Can you work these out from the model? Positions are in its coordinate system, mm. A direction names the side the tool comes from. Coordinates: 2 decimals unless noted, no trailing zeros. Order: outer loops, then holes, each group sorted by start corner. A loop starts at its lowest first (then second) coordinate and runs counter-clockwise, first axis right, second up. Notation, with made-up numbers: (37, -4) - (71, -4) arc R20 ccw to (71, 25) - close; hole circle Ø1 at (52.25, 71.25). An arc over 180 degrees is marked (long way). Use a Markdown table: item, result. Add a question column.
(1) I want a section at B-B (y = -5). List the corners of the cut face in (x, z) for me, and give its area (3 significant figures).
(2) If I drill on L1, parallel to Y at x = 16.5, z = -2; L2, parallel to Z at x = 3.5, y = 1.5; L3, parallel to Y at x = 6.5, z = -8.5, over which ranges is the centre line in solid material (lowest first)? Write a range as [from, to].
(3) On a 3-axis mill with a long thin cutter (end or side, diameter ignored), from which of +Z, -Z, +X, -X, +Y, -Y can I reach the whole of each face in a straight line? I mean faces 1 (the flat face through (16, -1, -6)), 2 (the cylindrical face through (0.8, -0.8, -5.6)), 3 (the flat face through (16, 0, -2)), 4 (the cylindrical face through (31.13, -0.84, -5.65)). Say none if no direction works.
(4) I want a section at A-A (x = 8). List the corners of the cut face in (y, z) for me, and give its area (3 significant figures).
(5) I want a section at C-C (z = -3.5). List the corners of the cut face in (x, y) for me, and give its area (3 significant figures).
(6) I want a section at D-D (y = 1). List the corners of the cut face in (x, z) for me.
(7) For pin 1 Ø1.4 at (x, z) = (10.5, -3.5) entering from -Y; pin 2 Ø4 at (x, y) = (18.5, -4.5) entering from +Z; pin 3 Ø2.5 at (x, z) = (23, -8.5) entering from +Y, each with a flat end and sliding along its axis, tell me the tip position at first contact or that it passes through.
```python
from build123d import *
from build123d.topology import SkipClean

# Parameters (mm, degrees)
BOSS_EXTRUDE1_DEPTH = 2
BOSS_EXTRUDE2_START = -7.6
BOSS_EXTRUDE2_DEPTH = 7.6
BOSS_EXTRUDE3_DEPTH = 2
SKETCH5_W           = 32
SKETCH5_H           = 4.6
CUT_EXTRUDE1_DEPTH  = 34.990586932


with BuildPart() as part:
    # Sketch1 → Boss-Extrude1 (new body)
    with BuildSketch(Plane(origin=(0, 0, 0), x_dir=(1, 0, 0), z_dir=(0, 1, 0))):
        with BuildLine():
            Line((2, 0), (30, 0))
            ThreePointArc((30, 0), (31.414213562, 0.585786438), (32, 2))
            Line((32, 2), (32, 4))
            ThreePointArc((32, 4), (31.414213562, 5.414213562), (30, 6))
            Line((30, 6), (2, 6))
            ThreePointArc((2, 6), (0.585786438, 5.414213562), (0, 4))
            Line((0, 4), (0, 2))
            ThreePointArc((0, 2), (0.585786438, 0.585786438), (2, 0))
        make_face()
    extrude(amount=BOSS_EXTRUDE1_DEPTH)

    # Sketch2 → Boss-Extrude2 (add)
    with SkipClean():  # the faces are left unmerged after this step: merging them gives an invalid solid
        with BuildSketch(Plane(origin=(0, 2, 0), x_dir=(1, 0, 0), z_dir=(0, 1, 0)).offset(BOSS_EXTRUDE2_START)):
            with BuildLine():
                Line((32, 4), (32, 2))
                ThreePointArc((32, 2), (31.449137675, 0.621595125), (30.1, 0.002501564))
                Line((30.1, 0.002501564), (30.1, 3.1))
                ThreePointArc((30.1, 3.1), (29.660660172, 4.160660172), (28.6, 4.6))
                Line((28.6, 4.6), (3.4, 4.6))
                ThreePointArc((3.4, 4.6), (2.339339828, 4.160660172), (1.9, 3.1))
                Line((1.9, 3.1), (1.9, 0.002501564))
                ThreePointArc((1.9, 0.002501564), (0.550862325, 0.621595125), (0, 2))
                Line((0, 2), (0, 4))
                ThreePointArc((0, 4), (0.585786438, 5.414213562), (2, 6))
                Line((2, 6), (30, 6))
                ThreePointArc((30, 6), (31.414213562, 5.414213562), (32, 4))
            make_face()
        extrude(amount=BOSS_EXTRUDE2_DEPTH)
    add(part.part.scale(1), mode=Mode.REPLACE)  # the faces are merged on a copy

    # Sketch4 → Boss-Extrude3 (add)
    with BuildSketch(Plane.XZ.offset(5.6)):
        with BuildLine():
            Line((30, -6), (2, -6))
            ThreePointArc((2, -6), (0.585786438, -5.414213562), (0, -4))
            Line((0, -4), (0, -8))
            ThreePointArc((0, -8), (0.585786438, -9.414213562), (2, -10))
            Line((2, -10), (30, -10))
            ThreePointArc((30, -10), (31.414213562, -9.414213562), (32, -8))
            Line((32, -8), (32, -4))
            ThreePointArc((32, -4), (31.414213562, -5.414213562), (30, -6))
        make_face()
    extrude(amount=-BOSS_EXTRUDE3_DEPTH)

    # Sketch5 → Cut-Extrude1 (cut, through all)
    with BuildSketch(Plane.XZ):
        with Locations((16, -2.3)):
            Rectangle(SKETCH5_W, SKETCH5_H)
    extrude(amount=CUT_EXTRUDE1_DEPTH, mode=Mode.SUBTRACT)


solid = part.part
```
Answers follow:
| question | item | result |
|---|---|---|
| 1 | outline | (0, -8) arc R2 ccw to (2, -10) - (30, -10) arc R2 ccw to (32, -8) - (32, -4.6) - (0, -4.6) - close |
| 1 | area | 171 mm² |
| 2 | L1 | y = [0, 2] |
| 2 | L2 | z = [-6, 0] |
| 2 | L3 | y = [-5.6, -3.6] |
| 3 | face 1 | -Z, +X, -X, +Y |
| 3 | face 2 | -Z, -X, +Y |
| 3 | face 3 | +Z, +X, -X, -Y |
| 3 | face 4 | -Z, +X, +Y |
| 4 | outline | (-5.6, -10) - (-3.6, -10) - (-3.6, -6) - (2, -6) - (2, 0) - (0, 0) - (0, -4.6) - (-5.6, -4.6) - close |
| 4 | area | 27.8 mm² |
| 5 | outline | (0, 0) - (32, 0) - (32, 2) - (0, 2) - close |
| 5 | area | 64.0 mm² |
| 6 | outline | (0, -4) arc R2 ccw to (2, -6) - (30, -6) arc R2 ccw to (32, -4) - (32, -2) arc R2 ccw to (30, 0) - (2, 0) arc R2 ccw to (0, -2) - close |
| 7 | pin 1 | stops at y = 0 |
| 7 | pin 2 | stops at z = -4.6 |
| 7 | pin 3 | stops at y = -3.6 |
